Design review of the part built by this model. Coordinates are the model's own, in mm. Face numbers are marked on the shaded views. A direction names the side the tool comes from. Give positions to 0.01 mm unless a question says otherwise; leave off trailing zeros. Loops run counter-clockwise (first coordinate to the right, second up) from the corner with the lowest first, then second, coordinate; pieces in that order, holes last. Notation, with made-up numbers: (53, -34) -> (93, -34) arc R32 cw to (93, 0) -> close; hole circle Ø7 at (29.5, 47.25). An arc over 180 degrees is marked (long way). Use CSV: the item, a comma, the result in double quotes. Start each with the question number.
Item 1: We need section D-D (x = 3.5). State the section outline as (y, z) points.
Item 2: We need section A-A (x = 12.7). State the section outline as (y, z) points.
Item 3: We need section C-C (z = -24). State the section outline as (x, y) points.
Item 4: The part is to be moulded in two halves that separate along X. For the marked faces 4, 5, 6 and 7, say which applies: +X half, -X half, draft (parallel to the pull), parting line (faces both ways), or undercut.
Item 5: We need section B-B (y = 10). State the section outline as (x, z) points, plus the area to 3 significant figures.
Item 6: Clearance check with flat-ended pins moving along their axes: pin 1 (2 mm diameter, centred on x = 15, y = 18, fed in from -Z); pin 2 (3.5 mm diameter, centred on x = 6.5, y = 16, fed in from +Z); pin 3 (4.5 mm diameter, centred on x = 7, z = 3, fed in from +Y). State where each tip first meets the part, or that it passes through.
Item 7: Wall thickness on line 1 along Y through (x, z) = (12.7, -26); line 2 along Z through (x, y) = (20.75, 3.5); line 3 along Y through (x, z) = (8.5, 1): over which ranges is each line inside the solid? List them lowest first. Write a range as from..to.
Item 8: For the marked faces 1, 2 and 3, list the 3-axis set-ups (+Z, -Z, +X, -X, +Y, -Y) from which the entire face can be reached by the end or side of a thin tool; tool diameter is ignored.
Autodesk Inventor part; units mm, degrees
ref_plane "YZ Plane" through (0, 0, 0) normal (1, 0, 0) x (0, 1, 0)
ref_plane "XZ Plane" through (0, 0, 0) normal (0, 1, 0) x (-1, 0, 0)
ref_plane "XY Plane" through (0, 0, 0) normal (0, 0, 1) x (1, 0, 0)
sketch "Sketch1" plane through (0, 0, 0) normal (1, 0, 0) x (0, 1, 0)
  line L0 (20, 0) -> (20, -40.0304)
  line L1 (20, -40.0304) -> (0, -40.0304)
  line L2 (0, -40.0304) -> (0, 0)
  line L3 (12.9972, 0) -> (7.0028, 0)
  line L4 (7.0028, 0) -> (7.0028, 5.5118)
  line L5 (7.0028, 5.5118) -> (12.9972, 5.5118)
  line L6 (12.9972, 5.5118) -> (12.9972, 0)
  line L7 (12.9972, -40.0304) -> (7.0028, -40.0304)
  line L8 (7.0028, -40.0304) -> (7.0028, -45.5422)
  line L9 (7.0028, -45.5422) -> (12.9972, -45.5422)
  line L10 (12.9972, -45.5422) -> (12.9972, -40.0304)
  line L11 (0, 0) -> (7.0028, 0)
  line L12 (12.9972, 0) -> (20, 0)
  dimension "d0" = 20
  dimension "d1" = 40.0304
  dimension "d2" = 5.5118
  dimension "d3" = 5.9944
  dimension "d4" = 5.5118
  dimension "d5" = 7.0028
  dimension "d6" = 7.0028
  dimension "d7" = 5.9944
extrude "Extrusion1" add sketch "Sketch1" along normal blind 25.4
sketch "Sketch2" plane through (0, 7.0028, 5.5118) normal (0, 0, 1) x (1, 0, 0)
  line L0 (0, 5.9944) -> (25.4, 5.9944)
  line L1 (25.4, 12.9972) -> (25.4, 5.9944)
  line L2 (0, 12.9972) -> (25.4, 12.9972)
  line L3 (0, 12.9972) -> (0, 5.9944)
  line L4 (0, 5.9944) -> (0, 0)
  line L5 (0, 0) -> (25.4, 0)
  line L6 (25.4, 5.9944) -> (25.4, 0)
  line L7 (0, 5.9944) -> (25.4, 5.9944)
  line L8 (0, 0) -> (25.4, 0)
  line L9 (0, 0) -> (0, -7.0028)
  line L10 (0, -7.0028) -> (25.4, -7.0028)
  line L11 (25.4, 0) -> (25.4, -7.0028)
  circle A0 centre (12.7, 2.9972) radius 2.54
  dimension "d10" = 5.08
extrude "Extrusion2" cut sketch "Sketch2" against normal blind 127 contours A0
equation "\"d4\" = d2"
equation "\"d5\" = 0.5 * d0 - 0.5 * d3"
equation "\"d6\" = d5"
equation "\"d7\" = d3"
properties part number "FrameSpacer"
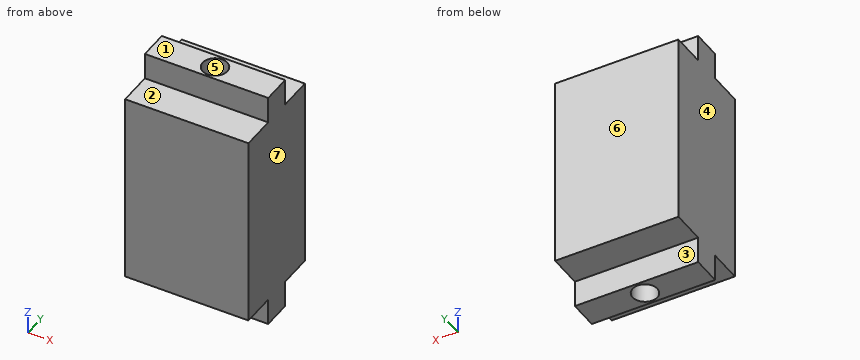
Results found:
1,outline,"(0, -40.03) -> (7, -40.03) -> (7, -45.54) -> (13, -45.54) -> (13, -40.03) -> (20, -40.03) -> (20, 0) -> (13, 0) -> (13, 5.51) -> (7, 5.51) -> (7, 0) -> (0, 0) -> close"
2,outline,"(0, -40.03) -> (7, -40.03) -> (7, -45.54) -> (7.46, -45.54) -> (7.46, 5.51) -> (7, 5.51) -> (7, 0) -> (0, 0) -> close; (12.54, -45.54) -> (13, -45.54) -> (13, -40.03) -> (20, -40.03) -> (20, 0) -> (13, 0) -> (13, 5.51) -> (12.54, 5.51) -> close"
3,outline,"(0, 0) -> (25.4, 0) -> (25.4, 20) -> (0, 20) -> close; hole circle Ø5.08 at (12.7, 10)"
4,face 4,"-X half"
4,face 5,"undercut"
4,face 6,"draft"
4,face 7,"+X half"
5,outline,"(0, -45.54) -> (10.16, -45.54) -> (10.16, 5.51) -> (0, 5.51) -> close; (15.24, -45.54) -> (25.4, -45.54) -> (25.4, 5.51) -> (15.24, 5.51) -> close"
5,area,"1,040 mm²"
6,pin 1,"z = -40.03"
6,pin 2,"z = 0"
6,pin 3,"y = 13"
7,line 1,"0..7.46, 12.54..20"
7,line 2,"-40.03..0"
7,line 3,"7..13"
8,face 1,"+Z, +X, -X, +Y, -Y"
8,face 2,"+Z, +X, -X, -Y"
8,face 3,"-Z, +X, -X, +Y"
